```python
from build123d import *

# Parameters (mm, degrees)
SKETCH1_R           = 2.25
EXTRUDE_1_DEPTH     = 10
SKETCH_1_R          = 21.25
CUT_EXTRUDE_1_DEPTH = 5
SKETCH_2_R          = 1.75
SKETCH_2_R_2        = 10
CUT_EXTRUDE_2_DEPTH = 5


with BuildPart() as part:
    # Sketch1 → 凸台-拉伸1 (new body)
    with BuildSketch(Plane(origin=(0, 0, 0), x_dir=(1, 0, 0), z_dir=(0, 1, 0))):
        with BuildLine():
            Line((-16.181288894, 69.127895164), (-14.556112863, 64.953423399))
            ThreePointArc((-14.556112863, 64.953423399), (0, 55), (14.556112863, 64.953423399))
            Line((14.556112863, 64.953423399), (16.181288894, 69.127895164))
            ThreePointArc((16.181288894, 69.127895164), (27.345655566, 75.32820205), (35.5, 65.5))
            Line((35.5, 65.5), (35.5, -65.5))
            ThreePointArc((35.5, -65.5), (27.345655566, -75.32820205), (16.181288894, -69.127895164))
            Line((16.181288894, -69.127895164), (14.556112863, -64.953423399))
            ThreePointArc((14.556112863, -64.953423399), (0, -55), (-14.556112863, -64.953423399))
            Line((-14.556112863, -64.953423399), (-16.181288894, -69.127895164))
            ThreePointArc((-16.181288894, -69.127895164), (-27.345655566, -75.32820205), (-35.5, -65.5))
            Line((-35.5, -65.5), (-35.5, 65.5))
            ThreePointArc((-35.5, 65.5), (-27.345655566, 75.32820205), (-16.181288894, 69.127895164))
        make_face()
        with Locations(Location((25.5, 65.5, 0), (0, 0, 270))):
            Circle(SKETCH1_R, mode=Mode.SUBTRACT)
        with Locations(Location((-25.5, 65.5, 0), (0, 0, 270))):
            Circle(SKETCH1_R, mode=Mode.SUBTRACT)
        with Locations(Location((-25.5, -65.5, 0), (0, 0, 270))):
            Circle(SKETCH1_R, mode=Mode.SUBTRACT)
        with Locations(Location((25.5, -65.5, 0), (0, 0, 270))):
            Circle(SKETCH1_R, mode=Mode.SUBTRACT)
    extrude(amount=EXTRUDE_1_DEPTH)

    # 草图1 → 切除-拉伸1 (cut)
    with BuildSketch(Plane(origin=(0, 10, 0), x_dir=(1, 0, 0), z_dir=(0, 1, 0))):
        with Locations(Location((0, 0, 0), (0, 0, 270))):
            Circle(SKETCH_1_R)
    extrude(amount=-CUT_EXTRUDE_1_DEPTH, mode=Mode.SUBTRACT)

    # 草图2 → 切除-拉伸2 (cut)
    with BuildSketch(Plane(origin=(0, 5, 0), x_dir=(1, 0, 0), z_dir=(0, 1, 0))):
        with Locations(Location((0, 14.5, 0), (0, 0, 270))):
            Circle(SKETCH_2_R)
        with Locations(Location((12.557368355, -7.25, 0), (0, 0, 270))):
            Circle(SKETCH_2_R)
        with Locations(Location((-12.557368355, -7.25, 0), (0, 0, 270))):
            Circle(SKETCH_2_R)
        with Locations(Location((0, 0, 0), (0, 0, 270))):
            Circle(SKETCH_2_R_2)
    extrude(amount=-CUT_EXTRUDE_2_DEPTH, mode=Mode.SUBTRACT)


solid = part.part
```
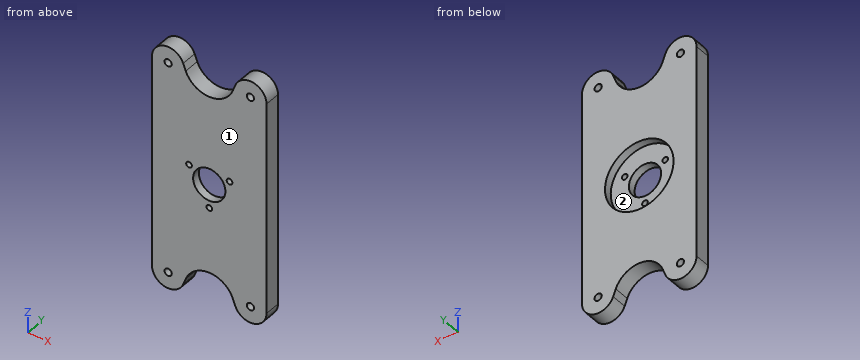
Source: CAD feature listing. Evaluate the final solid. Frame: model axes, mm. Face numbers are marked on the shaded views. Give positions to 0.01 mm unless a question says otherwise; leave off trailing zeros. Loops run counter-clockwise (first coordinate to the right, second up) from the corner with the lowest first, then second, coordinate; pieces in that order, holes last. Notation, with made-up numbers: (58, 8) - (71, 8) arc R17 cw to (71, 36) - close; hole circle Ø2 at (21.5, 81). An arc over 180 degrees is marked (long way). Use CSV: the item, a comma, the result in double quotes. Start each with the question number.
1. Section B-B (z = 0). Output: boundary loops of the cut face in (x, y), then the cut area to 4 significant figures.
2. Section A-A (x = 25.5). Output: boundary loops of the cut face in (y, z), then the cut area to 3 significant figures.
3. Section C-C (z = -60). Output: boundary loops of the cut face in (x, y), then the cut area to 3 significant figures.
4. Pin query (flat end, axial travel): pin 1 (2 mm diameter, centred on x = 1.5, y = 5.5, fed in from -Z); pin 2 (1 mm diameter, centred on x = 3, y = 7, fed in from +Z); pin 3 (1 mm diameter, centred on x = 24.5, y = 7.5, fed in from +Z). Return the tip coordinate at first contact, or that it passes through.
5. Draft query along Z for the marked faces 1 and 2. Return one class per face: +Z half, -Z half, draft (parallel to the pull), parting line (faces both ways), or undercut.
6. Ray query, L1, parallel to X at y = 3.3, z = 0; L2, parallel to Z at x = -26.5, y = 3.5; L3, parallel to X at y = 4, z = -65.5. Return the intervals inside material, ascending.
Response:
1,outline,"(-35.5, 0) - (-10, 0) - (-10, 5) - (-21.25, 5) - (-21.25, 10) - (-35.5, 10) - close; (10, 0) - (35.5, 0) - (35.5, 10) - (21.25, 10) - (21.25, 5) - (10, 5) - close"
1,area,"397.5 mm²"
2,outline,"(0, -75.5) - (10, -75.5) - (10, -67.75) - (0, -67.75) - close; (0, -63.25) - (10, -63.25) - (10, 63.25) - (0, 63.25) - close; (0, 67.75) - (10, 67.75) - (10, 75.5) - (0, 75.5) - close"
2,area,"1,420 mm²"
3,outline,"(-35.5, 0) - (-11.45, 0) - (-11.45, 10) - (-35.5, 10) - close; (11.45, 0) - (35.5, 0) - (35.5, 10) - (11.45, 10) - close"
3,area,"481 mm²"
4,pin 1,"z = -55.2"
4,pin 2,"z = 55.4"
4,pin 3,"z = 75.49"
5,face 1,"draft"
5,face 2,"undercut"
6,L1,"-35.5 to -10, 10 to 35.5"
6,L2,"-75.45 to -67.52, -63.48 to 63.48, 67.52 to 75.45"
6,L3,"-35.5 to -27.75, -23.25 to -14.77, 14.77 to 23.25, 27.75 to 35.5"
